Design review of the part built by this model. Coordinates are the model's own, in mm. Coordinates: 2 decimals unless noted, no trailing zeros. Loops run counter-clockwise (first coordinate to the right, second up) from the corner with the lowest first, then second, coordinate; pieces in that order, holes last. Notation, with made-up numbers: M 71.5,7 L 110.5,7 A19 ccw 110.5,39 Z; hole C 19,-39 d9. An arc over 180 degrees is marked long. Answer as a JSON object with one key per item and string values. Group by question number.
1. Draft analysis for pull direction Z (two halves, no side actions). For faces 1 (the flat face through (-14, 67, 57.249)), 2 (the cylindrical face through (-5.506, 66.731, -24.796)), 3 (the flat face through (-25, 135.358, 10)), state which applies: +Z half, -Z half, draft (parallel to the pull), parting line (faces both ways), or undercut.
2. Consider section B-B (z = 0). State the section outline as (x, y) points.
3. Consider section A-A (x = 0). State the section outline as (y, z) points, then the cut area to 3 significant figures.
4. Consider section C-C (y = 77). State the section outline as (x, z) points.
5. To check wall thickness, follow probe 1 along Z at (x, y) = (0, 74); probe 2 along Z at (x, y) = (-11, 124); probe 3 along X at (y, z) = (51.5, -7). State the ranges of each line that lie inside material, in increasing order.
from build123d import *

# Parameters (mm, degrees)
F0_W     = 102.013146
F0_H     = 95.492559
F0_R     = 25.4
F1_DEPTH = 135.357978


with BuildPart() as f1:
    # F0 (on Front) → F1 (new body)
    with BuildSketch(Plane.XZ):
        with Locations((-13.125478, 9.50263)):
            Rectangle(F0_W, F0_H)
        Circle(F0_R, mode=Mode.SUBTRACT)
    extrude(amount=-F1_DEPTH)


solid = f1.part
Findings below:
{
 "1": {"face 1": "+Z half", "face 2": "undercut", "face 3": "draft"},
 "2": {"outline": "M -64.13,0 L -25.4,0 L -25.4,135.36 L -64.13,135.36 Z; M 25.4,0 L 37.88,0 L 37.88,135.36 L 25.4,135.36 Z"},
 "3": {"outline": "M 0,-38.24 L 135.36,-38.24 L 135.36,-25.4 L 0,-25.4 Z; M 0,25.4 L 135.36,25.4 L 135.36,57.25 L 0,57.25 Z", "area": "6,050 mm^2"},
 "4": {"outline": "M -64.13,-38.24 L 37.88,-38.24 L 37.88,57.25 L -64.13,57.25 Z; hole C 0,0 d50.8"},
 "5": {"probe 1": "z = -38.24 to -25.4, 25.4 to 57.25", "probe 2": "z = -38.24 to -22.89, 22.89 to 57.25", "probe 3": "x = -64.13 to -24.42, 24.42 to 37.88"}
}
